Here's how the part is built. I have some questions about the finished solid (model axes, mm). A direction names the side the tool comes from. Round coordinates to 2 decimals unless told otherwise and drop trailing zeros. Write each loop counter-clockwise with the first axis right and the second up, starting at its lowest first coordinate (ties: lowest second). Pieces come first, ordered by that corner, then holes. Notation, with made-up numbers: M 22,-29.5 L 42,-29.5 A20 cw 42,-4.5 Z; hole C -9.75,74.25 d3. An arc over 180 degrees is marked long. Write item = value, one per line. Start each with the question number.
(1) Will these pins go through, and if not, where does the flat tip stop? pin 1 Ø10 at (x, y) = (-15, 8.5) entering from -Z; pin 2 Ø2 at (x, z) = (27.5, -6.5) entering from +Y; pin 3 Ø6 at (x, z) = (11.5, 1.5) entering from +Y; pin 4 Ø3.5 at (x, y) = (-16, 9.5) entering from +Z.
(2) On a 3-axis mill with a long thin cutter (end or side, diameter ignored), from which of +Z, -Z, +X, -X, +Y, -Y can I reach the whole of each face in a straight line? I mean faces 1 (the flat face through (1, 33.655, 25)), 2 (the flat face through (-1, 6.35, 23)), 3 (the flat face through (-1, 6.35, -24)). Say none if no direction works.
(3) I need wall thicknesses on line 1 along Z through (x, y) = (-16, 29); line 2 along Z through (x, y) = (-30.5, 13.5); line 3 along Y through (x, z) = (-7, -19). Which ranges of each line are inside material? Lowest first, please.
(4) I want a section at C-C (x = -5.5). List the corners of the cut face in (y, z) for me (3 decimals), and give its area (3 significant figures).
(5) I want a section at D-D (z = 0). List the corners of the cut face in (x, y) for me, and give its area (3 significant figures).
(6) If we mould it in two halves opening along Y, with no side actions, what happens to faces 4 (the flat face through (-38.1, 10, 0)), 5 (the flat face through (1, 33.655, -25)), 6 (the cylindrical face through (0.533, 20.656, 24.012))? For each: released by +Y, released by -Y, zero draft, split by the parting line, or undercut.
(7) I want a section at B-B (z = -24). List the corners of the cut face in (x, y) for me (3 decimals).
(8) I want a section at A-A (y = 29). List the corners of the cut face in (x, z) for me.
```python
from build123d import *

# Parameters (mm, degrees)
SKETCH1_W           = 76.2
SKETCH1_H           = 63.5
BOSS_EXTRUDE1_DEPTH = 6.35
BOSS_EXTRUDE2_DEPTH = 76.2
SKETCH3_W           = 30.48
SKETCH3_H           = 4.826
BOSS_EXTRUDE3_DEPTH = 76.2


with BuildPart() as part:
    # Sketch1 → Boss-Extrude1 (new body)
    with BuildSketch(Plane(origin=(0, 0, 0), x_dir=(1, 0, 0), z_dir=(0, 1, 0))):
        Rectangle(SKETCH1_W, SKETCH1_H)
    extrude(amount=BOSS_EXTRUDE1_DEPTH)



with BuildPart() as body_2:
    # Sketch2 → Boss-Extrude2 (new body)
    with BuildSketch(Plane(origin=(38.1, 0, 0), x_dir=(0, 0, -1), z_dir=(1, 0, 0))):
        with BuildLine():
            Line((-27.305, 33.655), (-22.225, 33.655))
            ThreePointArc((-22.225, 33.655), (0, 11.43), (22.225, 33.655))
            Line((22.225, 33.655), (27.305, 33.655))
            ThreePointArc((27.305, 33.655), (0, 6.35), (-27.305, 33.655))
        make_face()
    extrude(amount=-BOSS_EXTRUDE2_DEPTH)


with BuildPart() as part_1:
    add(part.part)

    add(body_2.part)  # Boss-Extrude3 merges body 2
    # Sketch3 → Boss-Extrude3 (add)
    with BuildSketch(Plane(origin=(38.1, 0, 0), x_dir=(0, 0, -1), z_dir=(1, 0, 0))):
        with Locations((0, 8.763)):
            Rectangle(SKETCH3_W, SKETCH3_H)
    extrude(amount=-BOSS_EXTRUDE3_DEPTH)


solid = part_1.part
```
Returned:
q1.pin_1 = -31.75
q1.pin_2 = 12.73
q1.pin_3 = 11.89
q1.pin_4 = 15.61
q2.face_1 = +Z, -Z, +X, -X, +Y
q2.face_2 = +Z, +X, -X
q2.face_3 = -Z, +X, -X
q3.line_1 = -26.91 to -21.73, 21.73 to 26.91
q3.line_2 = -18.42 to -9.37, 9.37 to 18.42
q3.line_3 = 0 to 6.35, 14.04 to 22.12
q4.outline = M 0,-31.75 L 6.35,-31.75 L 6.35,-15.24 L 10.999,-15.24 A27.305 ccw 33.655,-27.305 L 33.655,-22.225 A22.225 cw 33.655,22.225 L 33.655,27.305 A27.305 ccw 10.999,15.24 L 6.35,15.24 L 6.35,31.75 L 0,31.75 Z
q4.area = 844 mm²
q5.outline = M -38.1,0 L 38.1,0 L 38.1,11.43 L -38.1,11.43 Z
q5.area = 871 mm²
q6.face_4 = zero draft
q6.face_5 = released by +Y
q6.face_6 = undercut
q7.outline = M -38.1,0 L 38.1,0 L 38.1,6.35 L -38.1,6.35 Z; M -38.1,20.633 L 38.1,20.633 L 38.1,33.655 L -38.1,33.655 Z
q8.outline = M -38.1,-26.91 L 38.1,-26.91 L 38.1,-21.73 L -38.1,-21.73 Z; M -38.1,21.73 L 38.1,21.73 L 38.1,26.91 L -38.1,26.91 Z
